CAD build for the part. Positions are in the model's coordinates, mm. Face numbers are marked on the shaded views. Round coordinates to 2 decimals unless told otherwise and drop trailing zeros. Loops run counter-clockwise (first coordinate to the right, second up) from the corner with the lowest first, then second, coordinate; pieces in that order, holes last. Notation, with made-up numbers: M 47,22 L 66,22 A19 cw 66,55 Z; hole C 86.25,67 d7. An arc over 180 degrees is marked long. Put each result on its own line as item: value. Start each with the question number.
from build123d import *

# Parameters (mm, degrees)
SKETCH1_R           = 228.6
BOSS_EXTRUDE1_DEPTH = 168.91
FILLET1_R           = 22.86
SKETCH2_R           = 120.65
CUT_EXTRUDE1_DEPTH  = 127
FILLET2_R           = 20.32


with BuildPart() as part:
    # Sketch1 → Boss-Extrude1 (new body)
    with BuildSketch(Plane(origin=(0, 0, 0), x_dir=(1, 0, 0), z_dir=(0, 1, 0))):
        with Locations(Location((0, 0, 0), (0, 0, 270))):
            Circle(SKETCH1_R)
    extrude(amount=BOSS_EXTRUDE1_DEPTH)

    # Fillet1
    fillet1_edges = [part.edges().sort_by_distance(p)[0] for p in [
        (0, 0, -228.6),
        (0, 168.91, -228.6),
    ]]
    fillet(fillet1_edges, radius=FILLET1_R)

    # Sketch2 → Cut-Extrude1 (cut)
    with BuildSketch(Plane(origin=(0, 168.91, 0), x_dir=(1, 0, 0), z_dir=(0, 1, 0))):
        with Locations(Location((0, 0, 0), (0, 0, 270))):
            Circle(SKETCH2_R)
    extrude(amount=-CUT_EXTRUDE1_DEPTH, mode=Mode.SUBTRACT)

    # Fillet2
    fillet2_edges = [part.edges().sort_by_distance(p)[0] for p in [
        (0, 168.91, -120.65),
    ]]
    fillet(fillet2_edges, radius=FILLET2_R)


solid = part.part
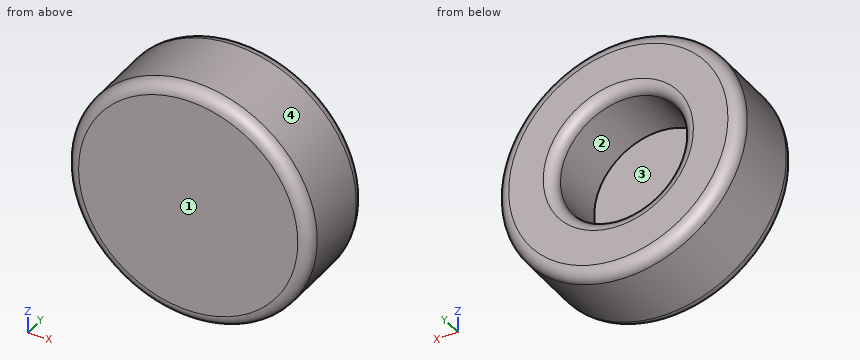
(1) Cut at C-C on y = 106. List the corners of the cut face in (x, z).
(2) Cut at B-B on z = 0. List the corners of the cut face in (x, y).
(3) Mould opens along X. For the marked faces 1, 2, 3 and 4 say: +X half, -X half, draft (parallel to the pull), parting line (faces both ways), or undercut.
(4) Cut at A-A on x = 0. List the corners of the cut face in (y, z).
(5) Drill centre lines: line 1 along X through (y, z) = (107, 0); line 2 along Y through (x, z) = (31.5, 112); line 3 along X through (y, z) = (73.5, -56). Where is each one in solid material? Low to high.
(6) Cut at D-D on y = 34.5. List the corners of the cut face in (x, z), and give its area (3 significant figures).
(7) Flat gauge pins, fed straight in: pin 1 Ø12 at (x, z) = (-97.5, -10) entering from -Y; pin 2 Ø8 at (x, y) = (85, 87.5) entering from -Z; pin 3 Ø2 at (x, z) = (135, -157) entering from +Y; pin 4 Ø1 at (y, z) = (44.5, -163) entering from +X. Where does each tip first touch, or does it go through?
Taken from the geometry:
1. outline: C 0,0 d457.2; hole C 0,0 d241.3
2. outline: M -228.6,22.86 A22.86 ccw -205.74,0 L 205.74,0 A22.86 ccw 228.6,22.86 L 228.6,146.05 A22.86 ccw 205.74,168.91 L 140.97,168.91 A20.32 ccw 120.65,148.59 L 120.65,41.91 L -120.65,41.91 L -120.65,148.59 A20.32 ccw -140.97,168.91 L -205.74,168.91 A22.86 ccw -228.6,146.05 Z
3. face 1: draft
3. face 2: undercut
3. face 3: undercut
3. face 4: parting line
4. outline: M 0,-205.74 A22.86 ccw 22.86,-228.6 L 146.05,-228.6 A22.86 ccw 168.91,-205.74 L 168.91,-140.97 A20.32 ccw 148.59,-120.65 L 41.91,-120.65 L 41.91,120.65 L 148.59,120.65 A20.32 ccw 168.91,140.97 L 168.91,205.74 A22.86 ccw 146.05,228.6 L 22.86,228.6 A22.86 ccw 0,205.74 Z
5. line 1: -228.6 to -120.65, 120.65 to 228.6
5. line 2: 0 to 41.91
5. line 3: -221.63 to -106.87, 106.87 to 221.63
6. outline: C 0,0 d457.2
6. area: 164,000 mm2
7. pin 1: y = 0
7. pin 2: z = -213.77
7. pin 3: y = 168.91
7. pin 4: x = 160.78
